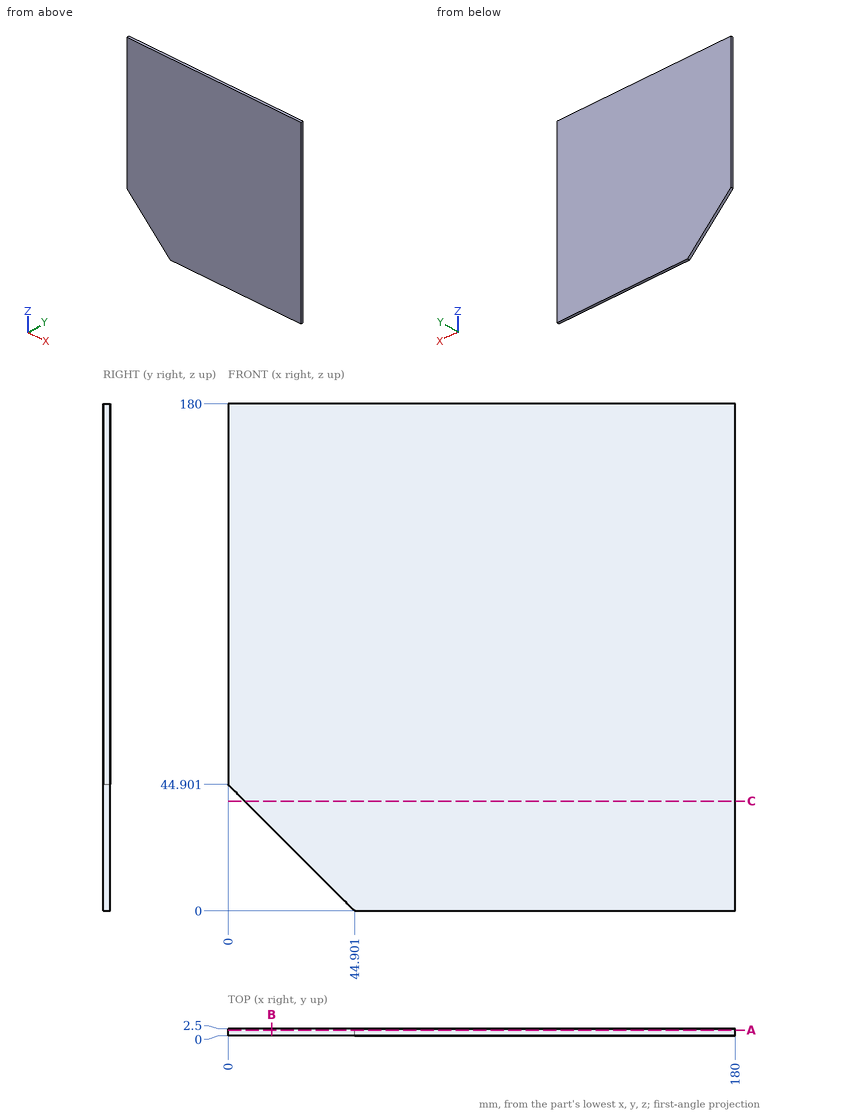
Answer from the drawing. Dimensions are ordinates in mm from the lowest x, y and z of the part. Give positions to 0.01 mm unless a question says otherwise; leave off trailing zeros. Order: outer loops, then holes, each group sorted by start corner. A loop starts at its lowest first (then second) coordinate and runs counter-clockwise, first axis right, second up.
(1) Find section A-A (y = 2.05). Give the vertices of the cut face in (x, z).
(2) Straight lines are drawn through the part: L1, parallel to Z at x = 31.5, y = 1.05; L2, parallel to Z at x = 44.5, y = 0.15; L3, parallel to X at y = 0.4, z = 12. For each, find the intervals that lie inside material, in ascending order.
(3) Find section C-C (z = 39). Give the vertices of the cut face in (x, y).
(4) Find section B-B (x = 15.5). Give the vertices of the cut face in (y, z).
Result sheet:
1. outline: (0, 44.9) - (44.9, 0) - (180, 0) - (180, 180) - (0, 180) - close
2. L1: z = 13.4 to 180
2. L2: z = 0.4 to 180
2. L3: x = 32.9 to 180
3. outline: (5.9, 0) - (180, 0) - (180, 2.5) - (5.9, 2.5) - close
4. outline: (0, 29.4) - (2.5, 29.4) - (2.5, 180) - (0, 180) - close
